Geometry check sheet. Reference: the model listing, model coordinates, mm. Give positions to 0.01 mm unless a question says otherwise; leave off trailing zeros. Loops run counter-clockwise (first coordinate to the right, second up) from the corner with the lowest first, then second, coordinate; pieces in that order, holes last.
Autodesk Inventor part; units mm, degrees
ref_plane "YZ Plane" through (0, 0, 0) normal (1, 0, 0) x (0, 1, 0)
ref_plane "XZ Plane" through (0, 0, 0) normal (0, 1, 0) x (-1, 0, 0)
ref_plane "XY Plane" through (0, 0, 0) normal (0, 0, 1) x (1, 0, 0)
sketch "Sketch1" plane through (0, 0, 0) normal (0, 0, 1) x (1, 0, 0)
  circle A0 centre (0, 0) radius 150
  circle A1 centre (0, 0) radius 100
  circle A2 centre (0, -125) radius 25
  circle A3 centre (73.4732, -101.1271) radius 25
  circle A4 centre (118.8821, -38.6271) radius 25
  circle A5 centre (118.8821, 38.6271) radius 25
  circle A6 centre (73.4732, 101.1271) radius 25
  circle A7 centre (0, 125) radius 25
  circle A8 centre (-73.4732, 101.1271) radius 25
  circle A9 centre (-118.8821, 38.6271) radius 25
  circle A10 centre (-118.8821, -38.6271) radius 25
  circle A11 centre (-73.4732, -101.1271) radius 25
  circle A12 centre (0, 0) radius 50
  circle A13 centre (0, 0) radius 155
  circle A14 centre (0, 0) radius 20
  circle A15 centre (20, 0) radius 2.5
  circle A16 centre (0, -20) radius 2.5
  circle A17 centre (-20, 0) radius 2.5
  circle A18 centre (0, 20) radius 2.5
  circle A19 centre (0, 0) radius 7
  circle A20 centre (0, 7) radius 1.6
  circle A21 centre (7, 0) radius 1.6
  circle A22 centre (0, -7) radius 1.6
  circle A23 centre (-7, 0) radius 1.6
  dimension "d0" = 300
  dimension "d1" = 200
  dimension "d2" = 50
  dimension "d5" = 360
  dimension "d7" = 100
  dimension "d13" = 310
  dimension "d17" = 40
  dimension "d18" = 5
  dimension "d19" = 5
  dimension "d20" = 5
  dimension "d21" = 5
  dimension "d29" = 14
  dimension "d30" = 3.2
  dimension "d31" = 3.2
  dimension "d32" = 3.2
  dimension "d33" = 3.2
extrude "Extrusion1" add sketch "Sketch1" along normal blind 5 contours A0 A4 A1 A5 | A5 A1 A6 A0 | A0 A3 A1 A4 | A6 A1 A7 A0 | A1 | A0 A2 A1 A3 | A7 A1 A8 A0 | A0 A11 A1 A2 | A8 A1 A9 A0 | A0 A10 A1 A11 | A9 A1 A10 A0 | A12 | A13 | A14 A15 | A14 A15 | A15 A14 A16 A17 A18 | A18 A14 | A14 A18 | A16 A14 | A14 A16 | A17 A14 | A14 A17 | A19 A21 | A19 A21 | A21 A19 A22 A23 A20 | A20 A19 | A19 A20 | A22 A19 | A19 A22 | A23 A19 | A19 A23
extrude "Extrusion5" cut sketch "Sketch1" along normal blind 5 contours A19 A21 | A19 A21 | A20 A19 | A19 A20 | A22 A19 | A19 A22 | A23 A19 | A19 A23
equation "\"d0\" = 6 * Product_dia"
equation "\"d1\" = 4 * Product_dia"
equation "\"d2\" = Product_dia"
equation "\"d7\" = 2 * Product_dia"
equation "\"Product_dia\" = 50"
equation "\"GridTotalSize\" = 63"
equation "\"GridBorderThickness\" = 5"
equation "\"GridBorderFillets\" = 7"
equation "\"BaseTotalWidth\" = 352"
equation "\"GridProcutClearance\" = 3"
equation "\"ProductBaseHeight\" = 35"
properties material "Acetal Resin, Black"
1) Sectioned sample at A-A on x = -112.5. Enter the section's corners in (y, z).
2) Scan lines: line 1 along Y through (x, z) = (0, 1.35); line 2 along Y through (x, z) = (-18.5, 3.7); line 3 along X through (y, z) = (-25, 2.35). Record each from-to range of solid material in increasing order.
3) Depth check by flat-ended pin: P1, Ø2.5, axis at x = 7, y = 0, coming from the +Z side; P2, Ø2, axis at y = -112, z = 1.5, coming from the -X side (3 decimals); P3, Ø1.5, axis at x = 94.5, z = 3.5, coming from the +Y side; P4, Ø3, axis at x = -41, z = 1.5, coming from the -Y side. Enter the tip coordinate at first touch or a pass-through.
4) Mould release check, pull along X, two halves, no side actions. Record for faces 1 (the flat face through (-2, 2, 0)), 2 (the cylindrical face through (-91.9, 84.23, 2.46)), 3 (the cylindrical face through (-33.601, 151.314, 2.465)): +X half, -X half, draft (parallel to the pull), parting line (faces both ways), or undercut.
5) Sectioned sample at C-C on z = 3.45. Count the separate pieces of the cut face and the enclosed holes in it, plus the area to 3 significant figures.
6) Sectioned sample at B-B on y = -60. Enter the section's corners in (x, z).
Determined:
1. outline: (-106.62, 0) - (-62.8, 0) - (-62.8, 5) - (-106.62, 5) - close; (-14.46, 0) - (14.46, 0) - (14.46, 5) - (-14.46, 5) - close; (62.8, 0) - (106.62, 0) - (106.62, 5) - (62.8, 5) - close
2. line 1: y = -155 to -150, -100 to -8.6, -5.4 to 5.4, 8.6 to 100, 150 to 155
2. line 2: y = -153.89 to -141.82, -108.18 to 108.18, 141.82 to 153.89
2. line 3: x = -152.97 to -139.84, -97.92 to 97.92, 139.84 to 152.97
3. P1: passes through
3. P2: stops at x = -108.185
3. P3: stops at y = 123.43
3. P4: stops at y = -149.88
4. face 1: draft
4. face 2: undercut
4. face 3: parting line
5. separate pieces: 1
5. enclosed holes: 14
5. area: 55,800 mm2
6. outline: (-142.92, 0) - (-131.85, 0) - (-131.85, 5) - (-142.92, 5) - close; (-105.91, 0) - (105.91, 0) - (105.91, 5) - (-105.91, 5) - close; (131.85, 0) - (142.92, 0) - (142.92, 5) - (131.85, 5) - close
